The figure shows three views and two pictorial views of one solid part (mm, origin at its lowest corner). Answer the questions. Round coordinates to 2 decimals unless told otherwise and drop trailing zeros. Order: outer loops, then holes, each group sorted by start corner. A loop starts at its lowest first (then second) coordinate and runs counter-clockwise, first axis right, second up. Notation, with made-up numbers: (-30.5, 56.25) - (-4.5, 56.25) arc R25 cw to (-4.5, 95.25) - close; hole circle Ø2 at (5, 25). An arc over 180 degrees is marked (long way). Answer in a Markdown table with one row per item.
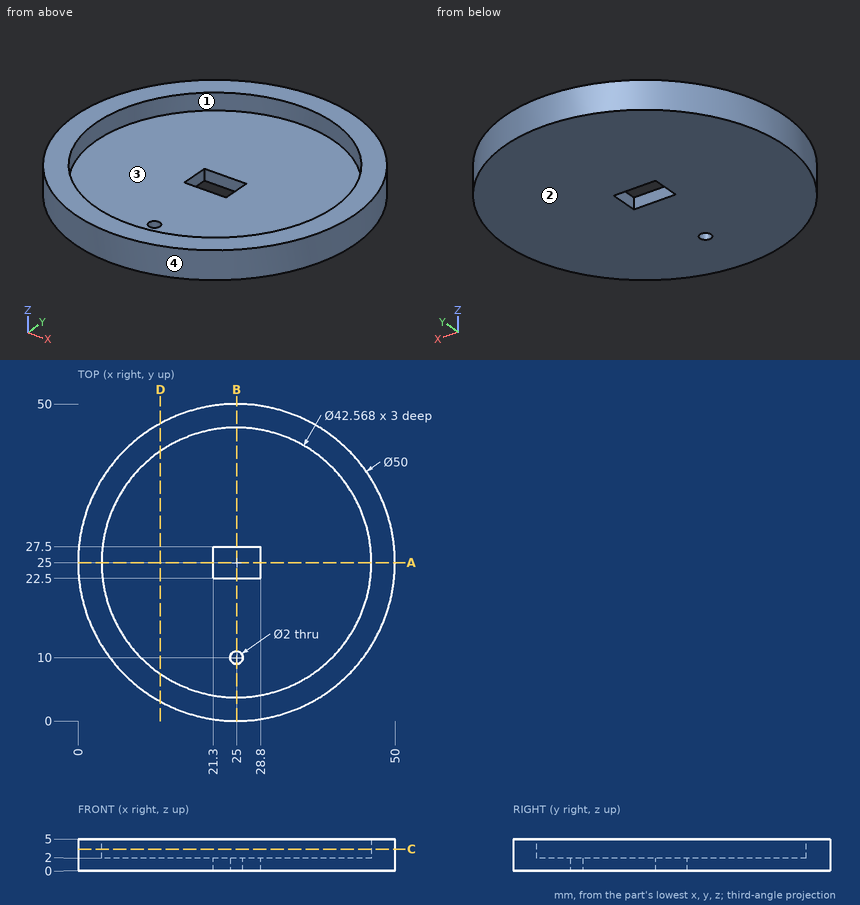
1) Find section C-C, the plane z = 3.4. Give the vertices of the cut face in (x, y).
Filled in:
| item | result |
|---|---|
| outline | circle Ø50 at (25, 25); hole circle Ø42.57 at (25, 25) |
2) Find the intervals of material crossed by probe 1 along Y at (x, z) = (25, 3.3); probe 2 along X at (y, z) = (25.5, 1.7) (3 decimals); probe 3 along Z at (x, y) = (20, 5), in increasing order. Write a range as from..to.
Filled in:
| item | result |
|---|---|
| probe 1 | y = 0..3.72, 46.28..50 |
| probe 2 | x = 0.005..21.3, 28.8..49.995 |
| probe 3 | z = 0..2 |
3) Find section D-D, the plane x = 13. Give the vertices of the cut face in (y, z).
Filled in:
| item | result |
|---|---|
| outline | (3.07, 0) - (46.93, 0) - (46.93, 5) - (42.58, 5) - (42.58, 2) - (7.42, 2) - (7.42, 5) - (3.07, 5) - close |
4) Find section A-A, the plane y = 25. Give the vertices of the cut face in (x, z).
Filled in:
| item | result |
|---|---|
| outline | (0, 0) - (21.3, 0) - (21.3, 2) - (3.72, 2) - (3.72, 5) - (0, 5) - close; (28.8, 0) - (50, 0) - (50, 5) - (46.28, 5) - (46.28, 2) - (28.8, 2) - close |
5) Find section B-B, the plane x = 25. Give the vertices of the cut face in (y, z).
Filled in:
| item | result |
|---|---|
| outline | (0, 0) - (9, 0) - (9, 2) - (3.72, 2) - (3.72, 5) - (0, 5) - close; (11, 0) - (22.5, 0) - (22.5, 2) - (11, 2) - close; (27.5, 0) - (50, 0) - (50, 5) - (46.28, 5) - (46.28, 2) - (27.5, 2) - close |
6) The mould has two halves that part along Y. Classify the marked faces 1, 2, 3 and 4: released by +Y, released by -Y, zero draft, split by the parting line, or undercut.
Filled in:
| item | result |
|---|---|
| face 1 | undercut |
| face 2 | zero draft |
| face 3 | undercut |
| face 4 | split by the parting line |
7) Each of these flat-tipped pins is pushed along its axis until it touches: pin 1 (2.5 mm diameter, centred on x = 25, y = 10, fed in from +Z); pin 2 (1 mm diameter, centred on x = 18, z = 4, fed in from -Y); pin 3 (1.5 mm diameter, centred on x = 43.5, z = 3.5, fed in from +Y) (1 decimal). Where does it stop, or does it pass through?
Filled in:
| item | result |
|---|---|
| pin 1 | stops at z = 2 |
| pin 2 | stops at y = 0.86 |
| pin 3 | stops at y = 42.6 |
